The model under review builds one solid part; all positions refer to its coordinate system, in mm. Face numbers are marked on the shaded views. Coordinates: 2 decimals unless noted, no trailing zeros. Order: outer loops, then holes, each group sorted by start corner. A loop starts at its lowest first (then second) coordinate and runs counter-clockwise, first axis right, second up. Notation, with made-up numbers: (-14.75, 76) -> (32.25, 76) arc R37 cw to (32.25, 112) -> close; hole circle Ø9 at (57.25, 27). An arc over 180 degrees is marked (long way). Use one line per item in the form item = value.
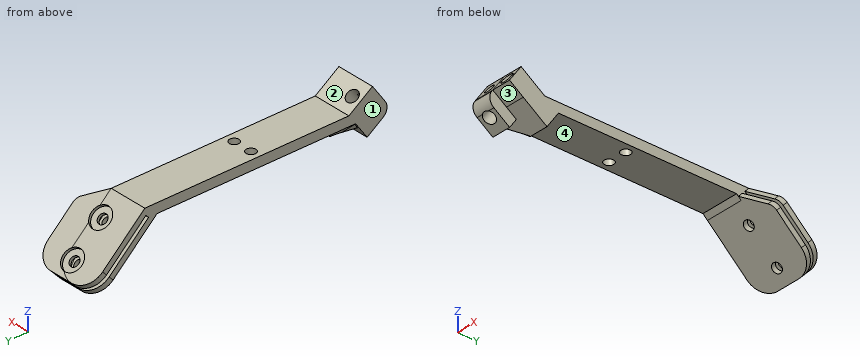
from build123d import *

# Parameters (mm, degrees)
BOSS_EXTRUDE1_DEPTH     = 20
CUT_EXTRUDE1_DEPTH      = 173.601162969
CUT_EXTRUDE1_DEPTH_BACK = 173.601162969
BOSS_EXTRUDE2_DEPTH     = 20
BOSS_EXTRUDE4_DEPTH     = 10
SKETCH7_R               = 3.1
CUT_EXTRUDE3_DEPTH      = 161.534558428
BOSS_EXTRUDE5_DEPTH     = 10
SKETCH9_R               = 3.1
CUT_EXTRUDE4_DEPTH      = 147.401949114
CUT_EXTRUDE5_DEPTH      = 175.168303714
CUT_EXTRUDE6_DEPTH      = 10
SKETCH12_R              = 2.5
CUT_EXTRUDE7_DEPTH      = 162.946023748
FILLET3_R               = 5
FILLET4_R               = 10
SKETCH15_R              = 2.5
CUT_EXTRUDE10_DEPTH     = 5
BOSS_EXTRUDE6_DEPTH     = 3
BOSS_EXTRUDE7_START     = -5
BOSS_EXTRUDE7_DEPTH     = 3
CUT_EXTRUDE11_REACH     = 164.653
SKETCH16_4_R            = 2.5
CHAMFER1_SIZE           = 8.3
FILLET5_R               = 5
SKETCH17_R              = 5.5
CUT_EXTRUDE12_DEPTH     = 1.5
FILLET6_R               = 5


# Read off the part's stored shape, not the designer's step: Save Bodies1
# Some blends are built 0.0001 mm under size
with BuildPart() as part:
    # Sketch1 → Boss-Extrude1 (new body)
    with BuildSketch(Plane(origin=(0, 0, 0), x_dir=(0, 0, -1), z_dir=(1, 0, 0))):
        Polygon((0, 0), (-27.279934402, -29.254148065), (-27.279934402, -169.254148065), (-22.279934402, -169.254148065), (-22.279934402, -31.223700443), (3.656768508, -3.4099918), align=None)
    extrude(amount=BOSS_EXTRUDE1_DEPTH)

    # Sketch2 → Cut-Extrude1 (cut, two sides: drawn at the far end of the back side and taken through both)
    with BuildSketch(Plane(origin=(20, 0, 0), x_dir=(0, 0, -1), z_dir=(1, 0, 0)).offset(-CUT_EXTRUDE1_DEPTH_BACK)):
        Polygon((2.194061105, -2.04599508), (-23.742641806, -29.859703723), (-22.279934402, -31.223700443), (3.656768508, -3.4099918), align=None)
    extrude(amount=CUT_EXTRUDE1_DEPTH + CUT_EXTRUDE1_DEPTH_BACK, mode=Mode.SUBTRACT)

    # Sketch3 → Boss-Extrude2 (add)
    with BuildSketch(Plane(origin=(20, 0, 0), x_dir=(0, 0, -1), z_dir=(1, 0, 0))):
        Polygon((3.656768508, -3.4099918), (-22.279934402, -31.223700443), (-20.085873298, -33.269695523), (5.850829613, -5.45598688), align=None)
        Polygon((-22.279934402, -35.622538), (-20.085873298, -33.269695523), (-22.279934402, -31.223700443), align=None)
    extrude(amount=-BOSS_EXTRUDE2_DEPTH)

    # Sketch6 → Boss-Extrude4 (add)
    with BuildSketch(Plane.ZY):
        Polygon((27.279934402, -135.441491542), (27.279934402, -153.753110374), (35.883580948, -147.728772207), align=None)
        Polygon((22.279934402, -138.942529233), (13.676287857, -144.9668674), (22.279934402, -157.254148065), align=None)
    extrude(amount=-BOSS_EXTRUDE4_DEPTH)

    # Sketch7 → Cut-Extrude3 (cut, through all)
    with BuildSketch(Plane(origin=(0, -41.266885928, -58.935220882), x_dir=(-1, 0, 0), z_dir=(0, -0.5735764363510402, -0.8191520442889961))):
        with Locations(Location((-5, -134.094302237, 0), (0, 0, 90))):
            Circle(SKETCH7_R)
    extrude(amount=-CUT_EXTRUDE3_DEPTH, mode=Mode.SUBTRACT)

    # Sketch8 → Boss-Extrude5 (add)
    with BuildSketch(Plane(origin=(20, 0, 0), x_dir=(0, 0, -1), z_dir=(1, 0, 0))):
        Polygon((-35.883580948, -147.728772207), (-31.581757675, -150.74094129), (-27.279934402, -144.597300958), (-27.279934402, -135.441491542), align=None)
        Polygon((-17.969117113, -131.300075805), (-22.279934402, -137.456560924), (-22.279934402, -146.61237034), (-13.695141582, -134.273766824), align=None)
        Polygon((-27.279934402, -144.597300958), (-31.581757675, -150.74094129), (-27.279934402, -153.753110374), align=None)
        Polygon((-22.279934402, -128.300751509), (-22.279934402, -137.456560924), (-17.969117113, -131.300075805), align=None)
    extrude(amount=-BOSS_EXTRUDE5_DEPTH)

    # Sketch9 → Cut-Extrude4 (cut, through all)
    with BuildSketch(Plane(origin=(0, -115.987262137, 81.215155285), x_dir=(-1, 0, 0), z_dir=(0, -0.8191520442889961, 0.5735764363510402))):
        with Locations(Location((-15, 60.591190556, 0), (0, 0, 90))):
            Circle(SKETCH9_R)
    extrude(amount=-CUT_EXTRUDE4_DEPTH, mode=Mode.SUBTRACT)

    # Sketch10 → Cut-Extrude5 (cut, through all)
    with BuildSketch(Plane.ZY):
        Polygon((22.279934402, -157.254148065), (27.279934402, -153.753110374), (27.279934402, -169.254148065), (22.279934402, -169.254148065), align=None)
    extrude(amount=-CUT_EXTRUDE5_DEPTH, mode=Mode.SUBTRACT)

    # Sketch11 → Cut-Extrude6 (cut)
    with BuildSketch(Plane(origin=(20, 0, 0), x_dir=(0, 0, -1), z_dir=(1, 0, 0))):
        Polygon((-22.279934402, -157.254148065), (-22.279934402, -146.61237034), (-27.279934403, -153.753110374), align=None)
    extrude(amount=-CUT_EXTRUDE6_DEPTH, mode=Mode.SUBTRACT)

    # Sketch12 → Cut-Extrude7 (cut, through all)
    with BuildSketch(Plane.XY.offset(27.279934402)):
        with Locations((5, -88.896520317)):
            Circle(SKETCH12_R)
        with Locations((15, -88.896520317)):
            Circle(SKETCH12_R)
    extrude(amount=-CUT_EXTRUDE7_DEPTH, mode=Mode.SUBTRACT)

    # Fillet3
    # the kernel refuses this fillet: 5 mm, written as the material it takes off along each edge
    with BuildSketch(Plane(origin=(-12.5, -157.254148065, 22.279934402), x_dir=(0, 0.5735764363510394, 0.8191520442889965), z_dir=(1, 0, 0))) as fillet3_piece_1:
        with BuildLine():
            CenterArc((FILLET3_R, -FILLET3_R), FILLET3_R, 90, 90)
            Line((0, -FILLET3_R), (0, 0))
            Line((0, 0), (FILLET3_R, 0))
        make_face()
    extrude(amount=35, mode=Mode.SUBTRACT)

    # Fillet4
    fillet4_edges = [part.edges().sort_by_distance(p)[0] for p in [
        (0, -4.43298934, -4.753799061),
        (20, -4.43298934, -4.753799061),
        (0, -1.02299754, -1.097030552),
        (20, -1.02299754, -1.097030552),
    ]]
    fillet(fillet4_edges, radius=FILLET4_R - 0.0001)  # a hair under: the kernel refuses the full size

    # Sketch15 → Cut-Extrude10 (cut)
    with BuildSketch(Plane(origin=(0, -115.987262137, 81.215155285), x_dir=(1, 0, 0), z_dir=(0, -0.8191520442889961, 0.5735764363510402))):
        with Locations(Location((5, -61.143127027, 0), (0, 0, 270))):
            Circle(SKETCH15_R)
    extrude(amount=-CUT_EXTRUDE10_DEPTH, mode=Mode.SUBTRACT)

    # Sketch16 → Boss-Extrude6 (add)
    with BuildSketch(Plane(origin=(0, 0, 0), x_dir=(1, 0, 0), z_dir=(0, 0.6819983600624997, 0.7313537016191695))):
        with BuildLine():
            Line((20, -10), (20, -40))
            Line((20, -40), (32.454585159, -30))
            Line((32.454585159, -30), (32.454585159, -10))
            ThreePointArc((32.454585159, -10), (29.52565297, -2.928932188), (22.454585159, 0))
            Line((22.454585159, 0), (10, 0))
            ThreePointArc((10, 0), (17.071067812, -2.928932188), (20, -10))
        make_face()
    extrude(amount=-BOSS_EXTRUDE6_DEPTH)

    # Sketch16<3> → Boss-Extrude7 (add)
    with BuildSketch(Plane(origin=(0, 0, 0), x_dir=(1, 0, 0), z_dir=(0, 0.6819983600624997, 0.7313537016191695)).offset(BOSS_EXTRUDE7_START)):
        with BuildLine():
            Line((20, -10), (20, -40))
            Line((20, -40), (32.454585159, -30))
            Line((32.454585159, -30), (32.454585159, -10))
            ThreePointArc((32.454585159, -10), (29.52565297, -2.928932188), (22.454585159, 0))
            Line((22.454585159, 0), (10, 0))
            ThreePointArc((10, 0), (17.071067812, -2.928932188), (20, -10))
        make_face()
    extrude(amount=-BOSS_EXTRUDE7_DEPTH)

    # Cut-Extrude11: up to this face of the body (flat: up to its plane)
    cut_extrude11_end = Plane(part.part.faces().sort_by_distance((15.482284505, -20.226716455, 7.923098549))[0])
    # Sketch16<4> → Cut-Extrude11 (cut, up to the picked face)
    with BuildSketch(Plane(origin=(0, 0, 0), x_dir=(1, 0, 0), z_dir=(0, 0.6819983600624997, 0.7313537016191695)), mode=Mode.PRIVATE) as cut_extrude11_sk1:
        with BuildLine():
            ThreePointArc((13.727292579, -8.030447622), (16.227292579, -10.530447622), (18.727292579, -8.030447622))
            Line((18.727292579, -8.030447622), (13.727292579, -8.030447622))
        make_face()
    cut_extrude11_tool1 = split(extrude(cut_extrude11_sk1.sketch, amount=-CUT_EXTRUDE11_REACH, mode=Mode.PRIVATE), bisect_by=cut_extrude11_end, keep=Keep.BOTH, mode=Mode.PRIVATE)
    # Sketch16<4> → Cut-Extrude11 (cut, up to the picked face)
    with BuildSketch(Plane(origin=(0, 0, 0), x_dir=(1, 0, 0), z_dir=(0, 0.6819983600624997, 0.7313537016191695)), mode=Mode.PRIVATE) as cut_extrude11_sk2:
        with BuildLine():
            Line((13.727292579, -8.030447622), (18.727292579, -8.030447622))
            ThreePointArc((18.727292579, -8.030447622), (16.227292579, -5.530447622), (13.727292579, -8.030447622))
        make_face()
    cut_extrude11_tool2 = split(extrude(cut_extrude11_sk2.sketch, amount=-CUT_EXTRUDE11_REACH, mode=Mode.PRIVATE), bisect_by=cut_extrude11_end, keep=Keep.BOTH, mode=Mode.PRIVATE)
    # Sketch16<4> → Cut-Extrude11 (cut, up to the picked face)
    with BuildSketch(Plane(origin=(0, 0, 0), x_dir=(1, 0, 0), z_dir=(0, 0.6819983600624997, 0.7313537016191695)), mode=Mode.PRIVATE) as cut_extrude11_sk3:
        with BuildLine():
            ThreePointArc((13.727292579, -8.030447622), (16.227292579, -10.530447622), (18.727292579, -8.030447622))
            Line((18.727292579, -8.030447622), (13.727292579, -8.030447622))
        make_face()
    cut_extrude11_tool3 = split(extrude(cut_extrude11_sk3.sketch, amount=-CUT_EXTRUDE11_REACH, mode=Mode.PRIVATE), bisect_by=cut_extrude11_end, keep=Keep.BOTH, mode=Mode.PRIVATE)
    # Sketch16<4> → Cut-Extrude11 (cut, up to the picked face)
    with BuildSketch(Plane(origin=(0, 0, 0), x_dir=(1, 0, 0), z_dir=(0, 0.6819983600624997, 0.7313537016191695)), mode=Mode.PRIVATE) as cut_extrude11_sk4:
        with BuildLine():
            Line((13.727292579, -8.030447622), (18.727292579, -8.030447622))
            ThreePointArc((18.727292579, -8.030447622), (16.227292579, -5.530447622), (13.727292579, -8.030447622))
        make_face()
    cut_extrude11_tool4 = split(extrude(cut_extrude11_sk4.sketch, amount=-CUT_EXTRUDE11_REACH, mode=Mode.PRIVATE), bisect_by=cut_extrude11_end, keep=Keep.BOTH, mode=Mode.PRIVATE)
    # Sketch16<4> → Cut-Extrude11 (cut, up to the picked face)
    with BuildSketch(Plane(origin=(0, 0, 0), x_dir=(1, 0, 0), z_dir=(0, 0.6819983600624997, 0.7313537016191695)), mode=Mode.PRIVATE) as cut_extrude11_sk5:
        with Locations(Location((16.227292579, -28.030447622, 0), (0, 0, 270))):
            Circle(SKETCH16_4_R)
    cut_extrude11_tool5 = split(extrude(cut_extrude11_sk5.sketch, amount=-CUT_EXTRUDE11_REACH, mode=Mode.PRIVATE), bisect_by=cut_extrude11_end, keep=Keep.BOTH, mode=Mode.PRIVATE)
    add(cut_extrude11_tool1.solids().sort_by(Axis((16.227293, -6.649088, 6.200375), (0, -0.6819983600624997, -0.7313537016191695)))[0], mode=Mode.SUBTRACT)
    add(cut_extrude11_tool2.solids().sort_by(Axis((16.227293, -5.097107, 4.753129), (0, -0.6819983600624997, -0.7313537016191695)))[0], mode=Mode.SUBTRACT)
    add(cut_extrude11_tool3.solids().sort_by(Axis((16.227293, -6.649088, 6.200375), (0, -0.6819983600624997, -0.7313537016191695)))[0], mode=Mode.SUBTRACT)
    add(cut_extrude11_tool4.solids().sort_by(Axis((16.227293, -5.097107, 4.753129), (0, -0.6819983600624997, -0.7313537016191695)))[0], mode=Mode.SUBTRACT)
    add(cut_extrude11_tool5.solids().sort_by(Axis((16.227293, -20.500172, 19.116719), (0, -0.6819983600624997, -0.7313537016191695)))[0], mode=Mode.SUBTRACT)

    # Chamfer1
    chamfer1_edges = [part.edges().sort_by_distance(p)[0] for p in [
        (10, -140.198799419, 20.485794641),
        (10, -133.621640371, 22.279934402),
    ]]
    chamfer(chamfer1_edges, length=CHAMFER1_SIZE)

    # Fillet5
    # the kernel refuses this fillet: 5 mm, written as the material it adds along each edge
    with BuildSketch(Plane(origin=(-1.165308952, -140.434114663, 25.145243354), x_dir=(-0.24426096127254496, -0.7383550160762786, -0.6286242542514651), z_dir=(0.6635786184004234, 0.34543716418991527, -0.6635786184004234))) as fillet5_piece_1_section:
        with BuildLine():
            CenterArc((FILLET5_R * 0.34543716419, FILLET5_R), FILLET5_R, 231.886370385, 38.113629615)
            Line((-FILLET5_R * 0.271785890905, FILLET5_R * 0.213211781824), (0, 0))
            Line((0, 0), (FILLET5_R * 0.34543716419, 0))
        make_face()
    fillet5_piece_1 = extrude(amount=21.143866778, mode=Mode.PRIVATE)
    fillet5_piece_1 = split(fillet5_piece_1, bisect_by=Plane(origin=(-1.165308952, -143.792687167, 20.318091976), z_dir=(0, 0.5711279895091977, 0.8208610233158727)), keep=Keep.TOP, mode=Mode.PRIVATE)
    fillet5_piece_1 = split(fillet5_piece_1, bisect_by=Plane(origin=(-1.165308952, -130.915194321, 18.522292961), z_dir=(0, -0.8208610233158725, 0.5711279895091982)), keep=Keep.TOP, mode=Mode.PRIVATE)
    fillet5_piece_1 = split(fillet5_piece_1, bisect_by=Plane(origin=(-1.165308952, -138.086990978, 23.501769657), z_dir=(0, 0.8191520442889962, -0.5735764363510399)), keep=Keep.TOP, mode=Mode.PRIVATE)
    add(fillet5_piece_1)

    # Sketch17 → Cut-Extrude12 (cut)
    with BuildSketch(Plane(origin=(0, 0, 0), x_dir=(1, 0, 0), z_dir=(0, 0.6819983600624997, 0.7313537016191695))):
        with Locations(Location((16.227292579, -28.030447622, 0), (0, 0, 270))):
            Circle(SKETCH17_R)
        with Locations(Location((16.227292579, -8.030447622, 0), (0, 0, 270))):
            Circle(SKETCH17_R)
    extrude(amount=-CUT_EXTRUDE12_DEPTH, mode=Mode.SUBTRACT)

    # Fillet6
    fillet6_edges = [part.edges().sort_by_distance(p)[0] for p in [
        (32.454585159, -22.963608589, 19.362920249),
        (32.454585159, -26.373600389, 15.706151741),
    ]]
    fillet(fillet6_edges, radius=FILLET6_R)


with BuildPart() as body_2:
    # Mirror1: mirrored copy
    add(part.part.mirror(Plane(origin=(30, 0, 0), x_dir=(0, 0, 1), z_dir=(1, 0, 0))))


solid = part.part
Item 1: Clearance check with flat-ended pins moving along their axes: pin 1 (5 mm diameter, centred on x = 21.5, z = 21, fed in from +Y); pin 2 (10 mm diameter, centred on x = 24.5, y = -113, fed in from +Z); pin 3 (6 mm diameter, centred on x = 28.5, z = 20, fed in from -Y); pin 4 (4.5 mm diameter, centred on x = 15, y = -88.9, fed in from -Z). State where each tip first meets the part, or that it passes through.
Results found:
pin_1 = -19.84
pin_2 = 27.28
pin_3 = -31.03
pin_4 = through
Item 2: Draft analysis for pull direction Y (two halves, no side actions). For the marked faces 1, 2, 3 and 4, state which applies: released by +Y, released by -Y, zero draft, split by the parting line, or undercut.
Results found:
face_1 = zero draft
face_2 = released by +Y
face_3 = released by -Y
face_4 = undercut
Item 3: We need section A-A (y = -117.5). Write out the cut boundary in (x, z).
Results found:
outline = (0, 22.28) -> (20, 22.28) -> (20, 27.28) -> (0, 27.28) -> close
Item 4: To check wall thickness, follow L1, parallel to Y at x = 5, z = 24; L2, parallel to Y at x = 15, z = 24; L3, parallel to Z at x = 3, y = -109.5. State the ranges of each line that lie inside material, in increasing order. Write a range as from..to.
Results found:
L1 = -155.27..-150.68, -143.11..-91.4, -86.4..-25.74
L2 = -149.07..-145.32, -134.51..-91.4, -86.4..-25.74
L3 = 22.28..27.28
